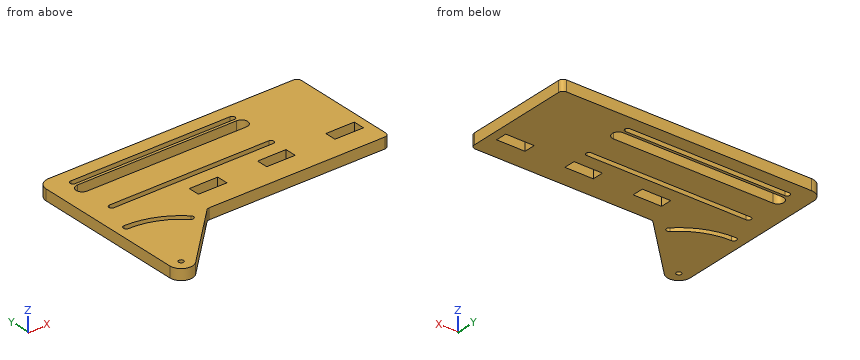
```python
from build123d import *

# Parameters (mm, degrees)
SKETCH1_R           = 1.3716
BOSS_EXTRUDE1_DEPTH = 6.0452
SKETCH2_W           = 15.875
SKETCH2_H           = 6.35
CUT_EXTRUDE1_DEPTH  = 6.0452
CUT_EXTRUDE2_DEPTH  = 7.62


with BuildPart() as part:
    # Sketch1 → Boss-Extrude1 (new body)
    with BuildSketch(Plane.XY):
        with BuildLine():
            Line((-6.35, 85.725), (-6.35, 0))
            ThreePointArc((-6.35, 0), (-2.430039796, -5.866635031), (4.490128061, -4.490128061))
            Line((4.490128061, -4.490128061), (31.430896424, 22.450640303))
            Line((31.430896424, 22.450640303), (36.811307345, 27.831051224))
            ThreePointArc((36.811307345, 27.831051224), (37.635342651, 28.381654013), (38.607358569, 28.575))
            Line((38.607358569, 28.575), (136.615256121, 28.575))
            ThreePointArc((136.615256121, 28.575), (138.411307345, 29.318948776), (139.155256121, 31.115))
            Line((139.155256121, 31.115), (139.155256121, 89.535))
            ThreePointArc((139.155256121, 89.535), (138.411307345, 91.331051224), (136.615256121, 92.075))
            Line((136.615256121, 92.075), (0, 92.075))
            ThreePointArc((0, 92.075), (-4.490128061, 90.215128061), (-6.35, 85.725))
        make_face()
        Circle(SKETCH1_R, mode=Mode.SUBTRACT)
        with BuildLine():
            ThreePointArc((25.818236348, 25.818236348), (13.972728824, 33.733151431), (0, 36.5125))
            ThreePointArc((0, 36.5125), (-1.5875, 38.1), (0, 39.6875))
            ThreePointArc((0, 39.6875), (15.187748722, 36.666468947), (28.063300378, 28.063300378))
            ThreePointArc((28.063300378, 28.063300378), (28.063300378, 25.818236348), (25.818236348, 25.818236348))
        make_face(mode=Mode.SUBTRACT)
    extrude(amount=BOSS_EXTRUDE1_DEPTH)

    # Sketch2 → Cut-Extrude1 (cut)
    with BuildSketch(Plane.XY.offset(6.0452)):
        with Locations((126.455256121, 43.815)):
            Rectangle(SKETCH2_W, SKETCH2_H)
        with Locations((88.355256121, 43.815)):
            Rectangle(SKETCH2_W, SKETCH2_H)
        with Locations((50.255256121, 43.815)):
            Rectangle(SKETCH2_W, SKETCH2_H)
    extrude(amount=-CUT_EXTRUDE1_DEPTH, mode=Mode.SUBTRACT)

    # Sketch3 → Cut-Extrude2 (cut)
    with BuildSketch(Plane(origin=(0, 0, 0), x_dir=(-1, 0, 0), z_dir=(0, 0, -1))):
        with BuildLine():
            Line((-95.25, 84.4804), (-6.35, 84.4804))
            ThreePointArc((-6.35, 84.4804), (-4.826, 82.9564), (-6.35, 81.4324))
            Line((-6.35, 81.4324), (-95.25, 81.4324))
            ThreePointArc((-95.25, 81.4324), (-96.774, 82.9564), (-95.25, 84.4804))
        make_face()
        with BuildLine():
            Line((-95.25, 57.6326), (-6.35, 57.6326))
            ThreePointArc((-6.35, 57.6326), (-4.826, 56.1086), (-6.35, 54.5846))
            Line((-6.35, 54.5846), (-95.25, 54.5846))
            ThreePointArc((-95.25, 54.5846), (-96.774, 56.1086), (-95.25, 57.6326))
        make_face()
        with BuildLine():
            Line((-95.25, 73.1266), (-6.35, 73.1266))
            ThreePointArc((-6.35, 73.1266), (-2.9464, 76.5302), (-6.35, 79.9338))
            Line((-6.35, 79.9338), (-95.25, 79.9338))
            ThreePointArc((-95.25, 79.9338), (-98.6536, 76.5302), (-95.25, 73.1266))
        make_face()
    extrude(amount=-CUT_EXTRUDE2_DEPTH, mode=Mode.SUBTRACT)


solid = part.part
```
Check sheet for the modelled part. Datum: model origin and axes. Units: mm. Round coordinates to 2 decimals unless told otherwise and drop trailing zeros. Loops run counter-clockwise (first coordinate to the right, second up) from the corner with the lowest first, then second, coordinate; pieces in that order, holes last. Notation, with made-up numbers: (27, -11.75) - (77, -11.75) arc R36 cw to (77, 24.25) - close; hole circle Ø10 at (19, 86.5). An arc over 180 degrees is marked (long way). Answer as a JSON object with one key per item and string values. Group by question number.
Q1. Sectioned sample at C-C, the plane y = 43.5. Enter the section's corners in (x, z).
Q2. Sectioned sample at A-A, the plane x = 82. Enter the section's corners in (y, z) (3 decimals), plus the area to 3 significant figures.
Q3. Scan lines: line 1 along Y through (x, z) = (74.5, 3.25) (3 decimals); line 2 along Y through (x, z) = (90.5, 1) (3 decimals); line 3 along X through (y, z) = (73.5, 0.75). Record each from-to range of solid material in increasing order. Write a range as [from, to].
Q4. Gauge pin test, flat ends, axial feed: P1, Ø3.5, axis at x = 0, y = 0, coming from the -Z side; P2, Ø1.8, axis at x = 91, z = 3, coming from the -Y side (3 decimals); P3, Ø5, axis at x = 53, y = 25, coming from the +Z side. Record the tip position at first contact, or that the pin passes through.
Q5. Sectioned sample at B-B, the plane x = 67. Enter the section's corners in (y, z) (3 decimals).
Q6. Sectioned sample at D-D, the plane x = 124.5. Enter the section's corners in (y, z) (3 decimals).
Solution:
{
 "1": {"outline": "(-6.35, 0) - (42.32, 0) - (42.32, 6.05) - (-6.35, 6.05) - close; (58.19, 0) - (80.42, 0) - (80.42, 6.05) - (58.19, 6.05) - close; (96.29, 0) - (118.52, 0) - (118.52, 6.05) - (96.29, 6.05) - close; (134.39, 0) - (139.16, 0) - (139.16, 6.05) - (134.39, 6.05) - close"},
 "2": {"outline": "(28.575, 0) - (40.64, 0) - (40.64, 6.045) - (28.575, 6.045) - close; (46.99, 0) - (54.585, 0) - (54.585, 6.045) - (46.99, 6.045) - close; (57.633, 0) - (73.127, 0) - (73.127, 6.045) - (57.633, 6.045) - close; (79.934, 0) - (81.432, 0) - (81.432, 6.045) - (79.934, 6.045) - close; (84.48, 0) - (92.075, 0) - (92.075, 6.045) - (84.48, 6.045) - close", "area": "267 mm²"},
 "3": {"line 1": "y = [28.575, 54.585], [57.633, 73.127], [79.934, 81.432], [84.48, 92.075]", "line 2": "y = [28.575, 40.64], [46.99, 54.585], [57.633, 73.127], [79.934, 81.432], [84.48, 92.075]", "line 3": "x = [-6.35, 4.8], [96.8, 139.16]"},
 "4": {"P1": "stops at z = 0", "P2": "stops at y = 28.575", "P3": "passes through"},
 "5": {"outline": "(28.575, 0) - (54.585, 0) - (54.585, 6.045) - (28.575, 6.045) - close; (57.633, 0) - (73.127, 0) - (73.127, 6.045) - (57.633, 6.045) - close; (79.934, 0) - (81.432, 0) - (81.432, 6.045) - (79.934, 6.045) - close; (84.48, 0) - (92.075, 0) - (92.075, 6.045) - (84.48, 6.045) - close"},
 "6": {"outline": "(28.575, 0) - (40.64, 0) - (40.64, 6.045) - (28.575, 6.045) - close; (46.99, 0) - (92.075, 0) - (92.075, 6.045) - (46.99, 6.045) - close"}
}
